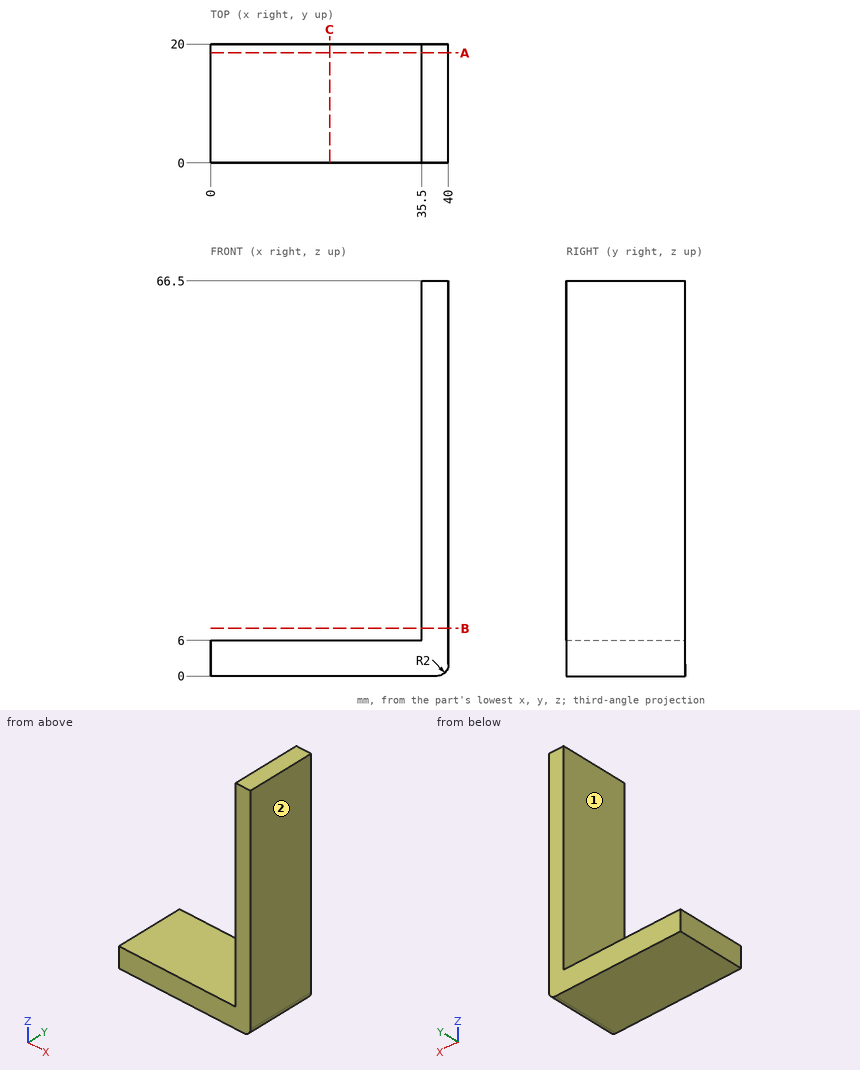
Could you check a few things on this drawing? It's one solid part, dimensions in mm from its lowest x, y, z. A direction names the side the tool comes from. Round coordinates to 2 decimals unless told otherwise and drop trailing zeros. Write each loop counter-clockwise with the first axis right and the second up, starting at its lowest first coordinate (ties: lowest second). Pieces come first, ordered by that corner, then holes. Notation, with made-up numbers: (74, 19) -> (125, 19) arc R15 ccw to (125, 40) -> close; hole circle Ø1 at (-25, 2.5). An arc over 180 degrees is marked (long way). Use a Markdown table: item, result.
1. Please list where these lines run through material, in increasing order: probe 1 along X at (y, z) = (15.5, 30.5); probe 2 along Z at (x, y) = (2, 18.25).
Answer key:
| item | result |
|---|---|
| probe 1 | x = 35.5 to 40 |
| probe 2 | z = 0 to 6 |
2. If we section it at B-B (z = 8): List the corners of the cut face in (x, y) for me, then the cut area to 3 significant figures.
Answer key:
| item | result |
|---|---|
| outline | (35.5, 0) -> (40, 0) -> (40, 20) -> (35.5, 20) -> close |
| area | 90.0 mm^2 |
3. If we section it at A-A (y = 18.5): List the corners of the cut face in (x, z) for me.
Answer key:
| item | result |
|---|---|
| outline | (0, 0) -> (38, 0) arc R2 ccw to (40, 2) -> (40, 66.5) -> (35.5, 66.5) -> (35.5, 6) -> (0, 6) -> close |
4. For pin 1 Ø10 at (x, y) = (10.5, 3.5) entering from +Z; pin 2 Ø5 at (y, z) = (7.5, 47) entering from -X, each with a flat end and sliding along its axis, tell me the tip position at first contact or that it passes through.
Answer key:
| item | result |
|---|---|
| pin 1 | stops at z = 6 |
| pin 2 | stops at x = 35.5 |
5. If we section it at C-C (x = 20): List the corners of the cut face in (y, z) for me, then the cut area to 3 significant figures.
Answer key:
| item | result |
|---|---|
| outline | (0, 0) -> (20, 0) -> (20, 6) -> (0, 6) -> close |
| area | 120 mm^2 |
6. Which directions (+Z, -Z, +X, -X, +Y, -Y) give clear straight access to the entire face, cutting with the end or side of a thin tool? Please do the marked faces 1 and 2.
Answer key:
| item | result |
|---|---|
| face 1 | +Z, -X, +Y, -Y |
| face 2 | +Z, -Z, +X, +Y, -Y |
